Verification items for the finished model (mm, model axes). A direction names the side the tool comes from. Give positions to 0.01 mm unless a question says otherwise; leave off trailing zeros. Loops run counter-clockwise (first coordinate to the right, second up) from the corner with the lowest first, then second, coordinate; pieces in that order, holes last. Notation, with made-up numbers: (29.25, 62) - (79.25, 62) arc R21 cw to (79.25, 94) - close; hole circle Ø9 at (-39.5, 1). An arc over 180 degrees is marked (long way). Answer in a Markdown table with one row per item.
```python
from build123d import *

# Parameters (mm, degrees)
SKETCH_1_W           = 57.5
SKETCH_1_H           = 100
EXTRUDE_1_DEPTH      = 3
SKETCH_2_R           = 2.6
CUT_EXTRUDE_1_DEPTH  = 0.8
SKETCH_3_R           = 1.25
CUT_EXTRUDE_2_DEPTH  = 58.754328842
SKETCH_3_3_R         = 2
CUT_EXTRUDE_3_DEPTH  = 1.5
EXTRUDE_2_DEPTH      = 3
SKETCH_5_3_W         = 57.5
SKETCH_5_3_H         = 3
SKETCH_5_3_W_2       = 2
EXTRUDE_3_DEPTH      = 29
SKETCH_6_W           = 8.2
SKETCH_6_H           = 3
CUT_EXTRUDE_4_DEPTH  = 3
CUT_EXTRUDE_START    = -3
SKETCH_6_4_R         = 0.35
CUT_EXTRUDE_6_DEPTH  = 3
SKETCH_7_W           = 3
SKETCH_7_H           = 10.666666667
EXTRUDE_4_DEPTH      = 3
FILLET_1_R           = 1.5
SKETCH_8_R           = 0.65
CUT_EXTRUDE_7_DEPTH  = 73.50215514
SKETCH_7_3_W         = 3
SKETCH_7_3_H         = 10.666666666
CUT_EXTRUDE_8_DEPTH  = 0.2
SKETCH_10_R          = 0.6
CUT_EXTRUDE_9_DEPTH  = 120.714504134
SKETCH_11_R          = 0.6
CUT_EXTRUDE_10_DEPTH = 93.03939374
SKETCH_12_R          = 1
CUT_EXTRUDE_11_DEPTH = 1.5
CUT_EXTRUDE_START_2  = -108.5
SKETCH_12_2_R        = 1
CUT_EXTRUDE_12_DEPTH = 1.5
SKETCH_13_R          = 1
CUT_EXTRUDE_13_DEPTH = 1.5


with BuildPart() as part:
    # 草图1 → 凸台-拉伸1 (new body)
    with BuildSketch(Plane(origin=(0, 0, 0), x_dir=(1, 0, 0), z_dir=(0, 1, 0))):
        Rectangle(SKETCH_1_W, SKETCH_1_H)
    extrude(amount=EXTRUDE_1_DEPTH)

    # 草图2 → 切除-拉伸1 (cut)
    with BuildSketch(Plane(origin=(0, 3, 0), x_dir=(1, 0, 0), z_dir=(0, 1, 0))):
        with Locations(Location((20.75, 43, 0), (0, 0, 270))):
            Circle(SKETCH_2_R)
        with Locations(Location((20.75, 12.5, 0), (0, 0, 270))):
            Circle(SKETCH_2_R)
        with Locations(Location((-20.75, 12.5, 0), (0, 0, 270))):
            Circle(SKETCH_2_R)
        with Locations(Location((-20.75, 43, 0), (0, 0, 270))):
            Circle(SKETCH_2_R)
    cut_extrude_1 = extrude(amount=-CUT_EXTRUDE_1_DEPTH, mode=Mode.SUBTRACT)

    # 草图3 → 切除-拉伸2 (cut, through all)
    with BuildSketch(Plane(origin=(0, 3, 0), x_dir=(1, 0, 0), z_dir=(0, 1, 0))):
        with Locations(Location((20.75, 27.75, 0), (0, 0, 270))):
            Circle(SKETCH_3_R)
        with Locations(Location((-20.75, 27.75, 0), (0, 0, 270))):
            Circle(SKETCH_3_R)
    cut_extrude_2 = extrude(amount=-CUT_EXTRUDE_2_DEPTH, mode=Mode.SUBTRACT)

    # 草图3<3> → 切除-拉伸3 (cut)
    with BuildSketch(Plane(origin=(0, 3, 0), x_dir=(1, 0, 0), z_dir=(0, 1, 0))):
        with Locations(Location((20.75, 27.75, 0), (0, 0, 270))):
            Circle(SKETCH_3_3_R)
        with Locations(Location((-20.75, 27.75, 0), (0, 0, 270))):
            Circle(SKETCH_3_3_R)
    cut_extrude_3 = extrude(amount=-CUT_EXTRUDE_3_DEPTH, mode=Mode.SUBTRACT)

    # 镜向1: 切除-拉伸1, 切除-拉伸2, 切除-拉伸3 across plane
    add(cut_extrude_1.mirror(Plane.XY), mode=Mode.SUBTRACT)
    add(cut_extrude_2.mirror(Plane.XY), mode=Mode.SUBTRACT)
    add(cut_extrude_3.mirror(Plane.XY), mode=Mode.SUBTRACT)

    # 草图5 → 凸台-拉伸2 (add)
    with BuildSketch(Plane(origin=(0, 3, 0), x_dir=(1, 0, 0), z_dir=(0, 1, 0))):
        Polygon((28.75, -50), (-28.75, -50), (-28.75, 50), (28.75, 50), (28.75, 55), (-34.75, 55), (-34.75, -55), (28.75, -55), align=None)
    extrude(amount=-EXTRUDE_2_DEPTH)

    # 草图5<3> → 凸台-拉伸3 (add)
    with BuildSketch(Plane(origin=(0, 3, 0), x_dir=(1, 0, 0), z_dir=(0, 1, 0))):
        with Locations((0, -53.5)):
            Rectangle(SKETCH_5_3_W, SKETCH_5_3_H)
        with Locations((0, 53.5)):
            Rectangle(SKETCH_5_3_W, SKETCH_5_3_H)
        Polygon((-30.75, -55), (-30.75, -52), (-30.75, 52), (-30.75, 55), (-34.75, 55), (-34.75, -55), align=None)
        with Locations((-29.75, 53.5)):
            Rectangle(SKETCH_5_3_W_2, SKETCH_5_3_H)
        with Locations((-29.75, -53.5)):
            Rectangle(SKETCH_5_3_W_2, SKETCH_5_3_H)
    extrude(amount=EXTRUDE_3_DEPTH)

    # 草图6 → 切除-拉伸4 (cut)
    with BuildSketch(Plane(origin=(28.75, 0, 0), x_dir=(0, 0, -1), z_dir=(1, 0, 0))):
        with Locations((0, 1.5)):
            Rectangle(SKETCH_6_W, SKETCH_6_H)
    extrude(amount=-CUT_EXTRUDE_4_DEPTH, mode=Mode.SUBTRACT)

    # 草图6<4> → 切除-拉伸6 (cut)
    with BuildSketch(Plane(origin=(28.75, 0, 0), x_dir=(0, 0, -1), z_dir=(1, 0, 0)).offset(CUT_EXTRUDE_START)):
        with Locations((0, 1.5)):
            Circle(SKETCH_6_4_R)
    extrude(amount=-CUT_EXTRUDE_6_DEPTH, mode=Mode.SUBTRACT)

    # 草图7 → 凸台-拉伸4 (add)
    with BuildSketch(Plane(origin=(28.75, 0, 0), x_dir=(0, 0, -1), z_dir=(1, 0, 0))):
        with Locations((-53.5, 26.666666666)):
            Rectangle(SKETCH_7_W, SKETCH_7_H)
        Polygon((-52, 10.666666667), (-55, 10.666666667), (-55, 0), (-52, 0), (-52, 3), align=None)
        with Locations((53.5, 26.666666666)):
            Rectangle(SKETCH_7_W, SKETCH_7_H)
        with Locations((53.5, 5.333333334)):
            Rectangle(SKETCH_7_W, SKETCH_7_H)
    extrude(amount=EXTRUDE_4_DEPTH)

    # 圆角1
    # the kernel refuses this fillet: 1.5 mm, written as the material it takes off along each edge
    with BuildSketch(Plane(origin=(31.75, 17.583333333, -55), x_dir=(-1, 0, 0), z_dir=(0, 1, 0)), Plane(origin=(31.75, 35.75, -52), x_dir=(-1, 0, 0), z_dir=(0, -1, 0)), Plane(origin=(31.75, -3.75, -55), x_dir=(-1, 0, 0), z_dir=(0, 1, 0)), Plane(origin=(31.75, 14.416666667, -52), x_dir=(-1, 0, 0), z_dir=(0, -1, 0)), Plane(origin=(31.75, 14.416666667, 55), x_dir=(-1, 0, 0), z_dir=(0, -1, 0)), Plane(origin=(31.75, 17.583333333, 52), x_dir=(-1, 0, 0), z_dir=(0, 1, 0)), Plane(origin=(31.75, 35.75, 55), x_dir=(-1, 0, 0), z_dir=(0, -1, 0))) as fillet_1_piece_1:
        with BuildLine():
            CenterArc((FILLET_1_R, FILLET_1_R), FILLET_1_R, 180, 90)
            Line((0, FILLET_1_R), (0, 0))
            Line((0, 0), (FILLET_1_R, 0))
        make_face()
    extrude(amount=18.166666667, mode=Mode.SUBTRACT)
    with BuildSketch(Plane(origin=(31.75, 14.416666667, 52), x_dir=(-1, 0, 0), z_dir=(0, -1, 0))) as fillet_1_piece_2:
        with BuildLine():
            CenterArc((FILLET_1_R, -FILLET_1_R), FILLET_1_R, 90, 90)
            Line((0, -FILLET_1_R), (0, 0))
            Line((0, 0), (FILLET_1_R, 0))
        make_face()
    extrude(amount=18.166666667, mode=Mode.SUBTRACT)

    # 草图8 → 切除-拉伸7 (cut, through all)
    with BuildSketch(Plane(origin=(0, 32, 0), x_dir=(1, 0, 0), z_dir=(0, 1, 0))):
        with Locations(Location((30.25, -53.5, 0), (0, 0, 270))):
            Circle(SKETCH_8_R)
        with Locations(Location((30.25, 53.5, 0), (0, 0, 270))):
            Circle(SKETCH_8_R)
    extrude(amount=-CUT_EXTRUDE_7_DEPTH, mode=Mode.SUBTRACT)

    # 草图7<3> → 切除-拉伸8 (cut)
    with BuildSketch(Plane(origin=(28.75, 0, 0), x_dir=(0, 0, -1), z_dir=(1, 0, 0))):
        with Locations((-53.5, 16)):
            Rectangle(SKETCH_7_3_W, SKETCH_7_3_H)
    extrude(amount=-CUT_EXTRUDE_8_DEPTH, mode=Mode.SUBTRACT)

    # 草图10 → 切除-拉伸9 (cut, through all)
    with BuildSketch(Plane(origin=(0, 0, -55), x_dir=(-1, 0, 0), z_dir=(0, 0, -1))):
        with Locations((-18.75, 30.5)):
            Circle(SKETCH_10_R)
        with Locations((1, 30.5)):
            Circle(SKETCH_10_R)
        with Locations((20.75, 30.5)):
            Circle(SKETCH_10_R)
    extrude(amount=-CUT_EXTRUDE_9_DEPTH, mode=Mode.SUBTRACT)

    # 草图11 → 切除-拉伸10 (cut, through all)
    with BuildSketch(Plane.ZY.offset(34.75)):
        with Locations((-34.6, 30.5)):
            Circle(SKETCH_11_R)
        with Locations((-17.3, 30.5)):
            Circle(SKETCH_11_R)
        with Locations((17.3, 30.5)):
            Circle(SKETCH_11_R)
        with Locations((34.6, 30.5)):
            Circle(SKETCH_11_R)
    extrude(amount=-CUT_EXTRUDE_10_DEPTH, mode=Mode.SUBTRACT)

    # 草图12 → 切除-拉伸11 (cut)
    with BuildSketch(Plane(origin=(0, 0, -55), x_dir=(-1, 0, 0), z_dir=(0, 0, -1))):
        with Locations((-18.75, 30.5)):
            Circle(SKETCH_12_R)
        with Locations((1, 30.5)):
            Circle(SKETCH_12_R)
        with Locations((20.75, 30.5)):
            Circle(SKETCH_12_R)
    extrude(amount=-CUT_EXTRUDE_11_DEPTH, mode=Mode.SUBTRACT)

    # 草图12<2> → 切除-拉伸12 (cut)
    with BuildSketch(Plane(origin=(0, 0, -55), x_dir=(-1, 0, 0), z_dir=(0, 0, -1)).offset(CUT_EXTRUDE_START_2)):
        with Locations((-18.75, 30.5)):
            Circle(SKETCH_12_2_R)
        with Locations((1, 30.5)):
            Circle(SKETCH_12_2_R)
        with Locations((20.75, 30.5)):
            Circle(SKETCH_12_2_R)
    extrude(amount=-CUT_EXTRUDE_12_DEPTH, mode=Mode.SUBTRACT)

    # 草图13 → 切除-拉伸13 (cut)
    with BuildSketch(Plane.ZY.offset(34.75)):
        with Locations((-34.6, 30.5)):
            Circle(SKETCH_13_R)
        with Locations((-17.3, 30.5)):
            Circle(SKETCH_13_R)
        with Locations((17.3, 30.5)):
            Circle(SKETCH_13_R)
        with Locations((34.6, 30.5)):
            Circle(SKETCH_13_R)
    extrude(amount=-CUT_EXTRUDE_13_DEPTH, mode=Mode.SUBTRACT)


solid = part.part
```
Q1. Go/stop test with flat-tipped pins: P1, Ø1.6, axis at x = -1, y = 30.5, coming from the +Z side; P2, Ø6, axis at x = 25, z = 26.5, coming from the +Y side; P3, Ø2, axis at x = -20, z = -28, coming from the +Y side. Record where each tip stops, or that it passes through.
Completed:
| item | result |
|---|---|
| P1 | z = 53.5 |
| P2 | y = 3 |
| P3 | y = 1.5 |
Q2. Sectioned sample at A-A (z = -27.75). Record the cut outline in (x, y).
Completed:
| item | result |
|---|---|
| outline | (-34.75, 0) - (-22, 0) - (-22, 1.5) - (-22.75, 1.5) - (-22.75, 3) - (-30.75, 3) - (-30.75, 32) - (-34.75, 32) - close; (-19.5, 0) - (19.5, 0) - (19.5, 1.5) - (18.75, 1.5) - (18.75, 3) - (-18.75, 3) - (-18.75, 1.5) - (-19.5, 1.5) - close; (22, 0) - (28.75, 0) - (28.75, 3) - (22.75, 3) - (22.75, 1.5) - (22, 1.5) - close |
Q3. Sectioned sample at D-D (z = -43). Record the cut outline in (x, y).
Completed:
| item | result |
|---|---|
| outline | (-34.75, 0) - (28.75, 0) - (28.75, 3) - (23.35, 3) - (23.35, 2.2) - (18.15, 2.2) - (18.15, 3) - (-18.15, 3) - (-18.15, 2.2) - (-23.35, 2.2) - (-23.35, 3) - (-30.75, 3) - (-30.75, 32) - (-34.75, 32) - close |
Q4. Sectioned sample at C-C (y = 16). Record the cut outline in (x, z).
Completed:
| item | result |
|---|---|
| outline | (-34.75, -55) - (28.75, -55) - (28.75, -52) - (-30.75, -52) - (-30.75, 52) - (28.55, 52) - (28.55, 55) - (-34.75, 55) - close |
Q5. Thickness scan on line 1 (Z direction, x = -20.5, y = 13.5); line 2 (X direction, y = 2.5, z = -27.75); line 3 (Z direction, x = -20, y = 2). Record the ranges inside material, lowest first.
Completed:
| item | result |
|---|---|
| line 1 | -55 to -52, 52 to 55 |
| line 2 | -34.75 to -22.75, -18.75 to 18.75, 22.75 to 28.75 |
| line 3 | -55 to -29.6, -25.9 to 25.9, 29.6 to 55 |
Q6. Tool access check on faces 3 (the face through (-1, 16, 52)), 4 (the face through (-20.62, 31.49, -54.26)), 5 (the face through (-34.01, 31.49, 17.17)), 6 (the face through (22.94, 2.61, 11.1)), 7 (the face through (27, 1, -4.1)). Record the directions out of +Z, -Z, +X, -X, +Y, -Y that give a thin tool (end or side, any length) a straight path to the whole face; none if there is none.
Completed:
| item | result |
|---|---|
| face 3 | +X, +Y |
| face 4 | -Z |
| face 5 | -X |
| face 6 | +Y |
| face 7 | +X, +Y, -Y |
Q7. Sectioned sample at B-B (y = 28). Record the cut outline in (x, z).
Completed:
| item | result |
|---|---|
| outline | (-34.75, -55) - (30.25, -55) arc R1.5 ccw to (30.25, -52) - (-30.75, -52) - (-30.75, 52) - (30.25, 52) arc R1.5 ccw to (30.25, 55) - (-34.75, 55) - close; hole circle Ø1.3 at (30.25, -53.5); hole circle Ø1.3 at (30.25, 53.5) |
Q8. Draft check along Z on faces 1 (the face through (-34.75, 16, -1)), 2 (the face through (31.75, 26.74, 53.47)). Enter one of: +Z half, -Z half, draft (parallel to the pull), parting line (faces both ways), or undercut.
Completed:
| item | result |
|---|---|
| face 1 | draft |
| face 2 | undercut |
